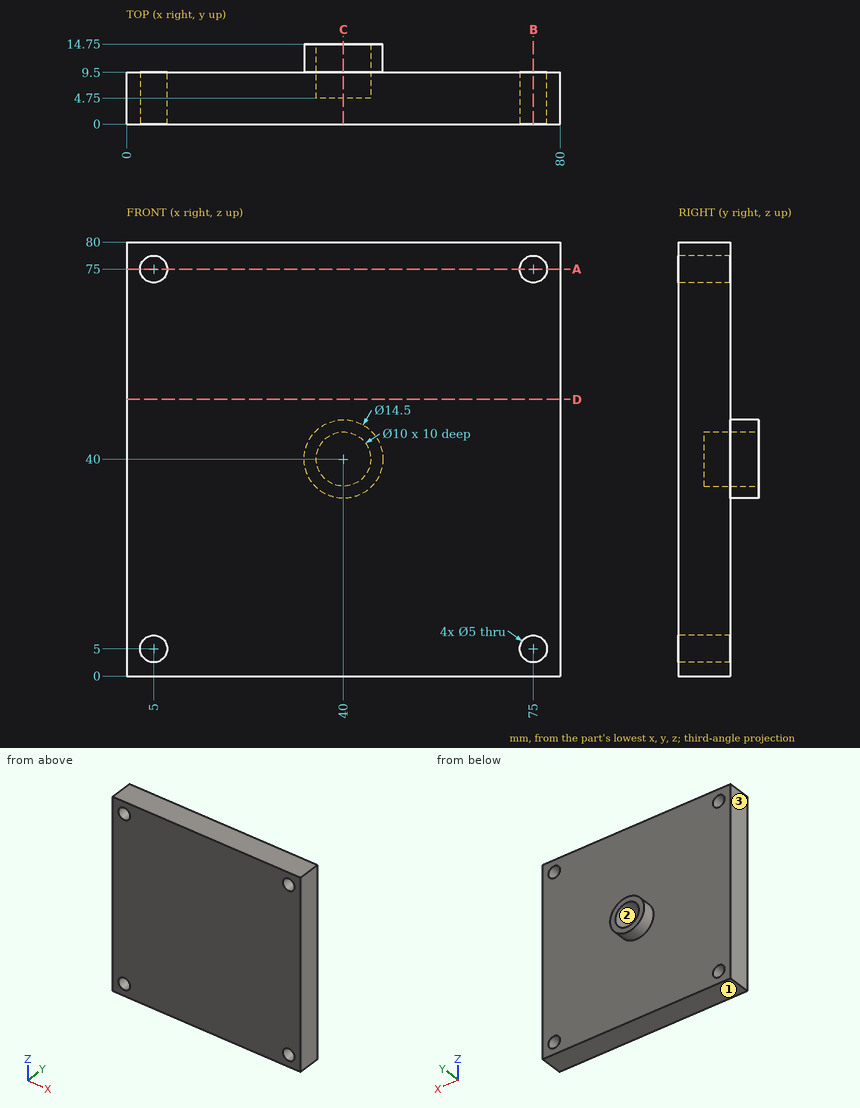
Verification items for this drawing (mm, ordinates from the low corner). Give positions to 0.01 mm unless a question says otherwise; leave off trailing zeros. Write each loop counter-clockwise with the first axis right and the second up, starting at its lowest first coordinate (ties: lowest second). Pieces come first, ordered by that corner, then holes. Notation, with made-up numbers: (64.5, 73) -> (122.5, 73) arc R17 cw to (122.5, 103) -> close; hole circle Ø10 at (-21.75, 76.5). An arc over 180 degrees is marked (long way). Use CSV: the item, a comma, the result in double quotes.
(1) Go/stop test with flat-tipped pins: pin 1 (8 mm diameter, centred on x = 5, z = 5, fed in from +Y); pin 2 (5 mm diameter, centred on x = 29, z = 57.5, fed in from -Y). Record where each tip stops, or that it passes through.
Derived:
pin 1,"stops at y = 9.5"
pin 2,"stops at y = 0"
(2) Sectioned sample at A-A (z = 75). Record the cut outline in (x, y), plus the area to 3 significant figures.
Derived:
outline,"(0, 0) -> (2.5, 0) -> (2.5, 9.5) -> (0, 9.5) -> close; (7.5, 0) -> (72.5, 0) -> (72.5, 9.5) -> (7.5, 9.5) -> close; (77.5, 0) -> (80, 0) -> (80, 9.5) -> (77.5, 9.5) -> close"
area,"665 mm^2"
(3) Sectioned sample at B-B (x = 75). Record the cut outline in (y, z).
Derived:
outline,"(0, 0) -> (9.5, 0) -> (9.5, 2.5) -> (0, 2.5) -> close; (0, 7.5) -> (9.5, 7.5) -> (9.5, 72.5) -> (0, 72.5) -> close; (0, 77.5) -> (9.5, 77.5) -> (9.5, 80) -> (0, 80) -> close"
(4) Material ranges on L1, parallel to X at y = 2.5, z = 5; L2, parallel to Z at x = 40, y = 12, recorded low to high.
Derived:
L1,"x = 0 to 2.5, 7.5 to 72.5, 77.5 to 80"
L2,"z = 32.75 to 35, 45 to 47.25"
(5) Sectioned sample at C-C (x = 40). Record the cut outline in (y, z), plus the area to 3 significant figures.
Derived:
outline,"(0, 0) -> (9.5, 0) -> (9.5, 32.75) -> (14.75, 32.75) -> (14.75, 35) -> (4.75, 35) -> (4.75, 45) -> (14.75, 45) -> (14.75, 47.25) -> (9.5, 47.25) -> (9.5, 80) -> (0, 80) -> close"
area,"736 mm^2"
(6) Sectioned sample at D-D (z = 51). Record the cut outline in (x, y), plus the area to 3 significant figures.
Derived:
outline,"(0, 0) -> (80, 0) -> (80, 9.5) -> (0, 9.5) -> close"
area,"760 mm^2"
(7) Release check for a two-part mould opening along Z. For the marked faces 1, 2 and 3 record: +Z half, -Z half, draft (parallel to the pull), parting line (faces both ways), or undercut.
Derived:
face 1,"-Z half"
face 2,"undercut"
face 3,"draft"
